Design review of the part built by this model. Coordinates are the model's own, in mm. Face numbers are marked on the shaded views. A direction names the side the tool comes from. Round coordinates to 2 decimals unless told otherwise and drop trailing zeros. Order: outer loops, then holes, each group sorted by start corner. A loop starts at its lowest first (then second) coordinate and runs counter-clockwise, first axis right, second up. Notation, with made-up numbers: (64.5, 50) - (76.5, 50) arc R21 cw to (76.5, 59) - close; hole circle Ø6 at (20.25, 70.5). An arc over 180 degrees is marked (long way). Use CSV: the item, a comma, the result in double quotes. Start each with the question number.
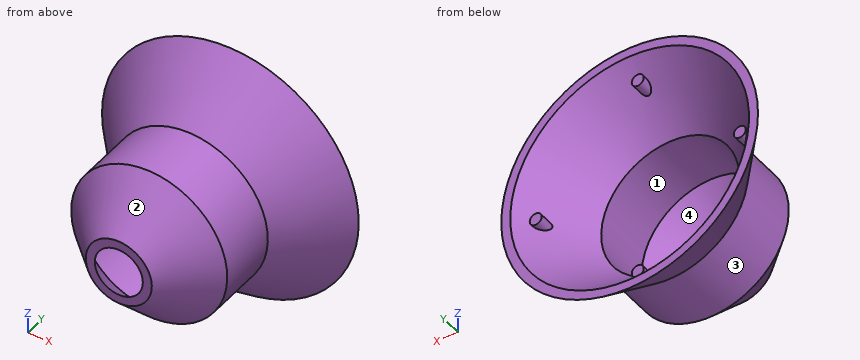
from build123d import *

# Parameters (mm, degrees)
SKETCH1_R           = 13
SKETCH1_R_2         = 11.5
BOSS_EXTRUDE1_DEPTH = 10
BOSS_EXTRUDE2_REACH = 40.265
BOSS_EXTRUDE2_START = -2
SKETCH5_R           = 1
CIRPATTERN1_COUNT   = 4


with BuildPart() as part:
    # Sketch1 → Boss-Extrude1 (new body)
    with BuildSketch(Plane(origin=(0, 0, 0), x_dir=(1, 0, 0), z_dir=(0, 1, 0))):
        with Locations(Location((0, 0, 0), (0, 0, 270))):
            Circle(SKETCH1_R)
        with Locations(Location((0, 0, 0), (0, 0, 270))):
            Circle(SKETCH1_R_2, mode=Mode.SUBTRACT)
    extrude(amount=BOSS_EXTRUDE1_DEPTH)

    # Sketch4 → Revolve1 (revolve)
    with BuildSketch(Plane.XY, mode=Mode.PRIVATE) as revolve1_sk:
        Polygon((-13, 10), (-21.390996312, 20), (-19.890996312, 20), (-11.5, 10), align=None)
    revolve(revolve1_sk.sketch.rotate(Axis((0, 18.930839499, 0), (0, -1, 0)), 270), axis=Axis((0, 18.930839499, 0), (0, -1, 0)))

    # Sketch5 → Boss-Extrude2 (add, up to next)
    with BuildSketch(Plane(origin=(0, 20, 0), x_dir=(1, 0, 0), z_dir=(0, 1, 0)).offset(BOSS_EXTRUDE2_START), mode=Mode.PRIVATE) as boss_extrude2_sk1:
        with Locations(Location((-17, 0, 0), (0, 0, 270))):
            Circle(SKETCH5_R)
    boss_extrude2_tool1 = extrude(boss_extrude2_sk1.sketch, amount=-BOSS_EXTRUDE2_REACH, mode=Mode.PRIVATE) - part.part
    boss_extrude2 = boss_extrude2_tool1.solids().sort_by_distance((-17, 18, 0))[0]
    add(boss_extrude2)

    # CirPattern1: Boss-Extrude2 ×4 about axis
    cirpattern1_axis = Axis((0, 0, 0), (0, 1, 0))
    for i in range(1, CIRPATTERN1_COUNT):
        add(boss_extrude2.rotate(cirpattern1_axis, i * 360 / CIRPATTERN1_COUNT))

    # Sketch6 → Revolve2 (revolve)
    with BuildSketch(Plane.XY, mode=Mode.PRIVATE) as revolve2_sk:
        Polygon((-13, 0), (-5.5, -7.5), (-4, -7.5), (-11.5, 0), align=None)
    revolve(revolve2_sk.sketch.rotate(Axis((0, 18.930839499, 0), (0, -1, 0)), 270), axis=Axis((0, 18.930839499, 0), (0, -1, 0)))


solid = part.part
Q1. The part is to be moulded in two halves that separate along X. For the marked faces 1 and 2, say which applies: +X half, -X half, draft (parallel to the pull), parting line (faces both ways), or undercut.
Q2. Tool access review of the marked faces 3 and 4: name each direction out of +Z, -Z, +X, -X, +Y, -Y from which nothing blocks a thin tool from reaching the whole face with its end or side.
Q3. Take a section at A-A (z = 0). State the section outline as (x, y) points.
Q4. For L1, parallel to X at y = 2.75, z = 0; L2, parallel to Z at x = -0.5, y = 6.5; L3, parallel to X at y = 13, z = 10, list the stretches that pass through material, from the lowest coordinate up. Write a range as [from, to].
Q5. Clearance check with flat-ended pins moving along their axes: pin 1 (2 mm diameter, centred on x = 0.5, z = 17, fed in from +Y); pin 2 (1.5 mm diameter, centred on x = -14.5, z = 1.5, fed in from -Y); pin 3 (10 mm diameter, centred on y = 8.5, z = 10.5, fed in from +X). State where each tip first meets the part, or that it passes through.
Findings below:
1,face 1,"undercut"
1,face 2,"parting line"
2,face 3,"-Y"
2,face 4,"+Y"
3,outline,"(-21.39, 20) - (-13, 10) - (-13, 0) - (-5.5, -7.5) - (-4, -7.5) - (-11.5, 0) - (-11.5, 10) - (-16, 15.36) - (-16, 18) - (-18, 18) - (-18, 17.75) - (-19.89, 20) - close; (4, -7.5) - (5.5, -7.5) - (13, 0) - (13, 10) - (21.39, 20) - (19.89, 20) - (18, 17.75) - (18, 18) - (16, 18) - (16, 15.36) - (11.5, 10) - (11.5, 0) - close"
4,L1,"x = [-13, -11.5], [11.5, 13]"
4,L2,"z = [-12.99, -11.49], [11.49, 12.99]"
4,L3,"x = [-11.87, -9.82], [9.82, 11.87]"
5,pin 1,"stops at y = 18"
5,pin 2,"stops at y = 10.99"
5,pin 3,"stops at x = 13.13"
